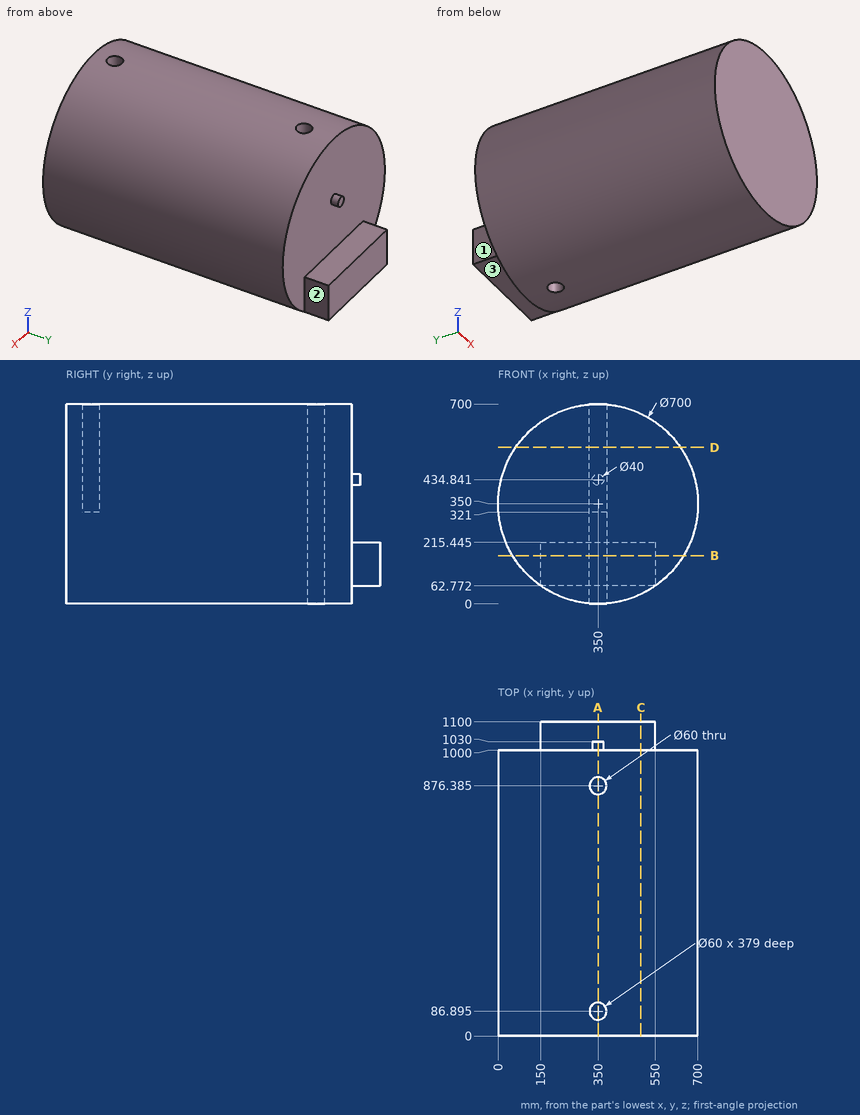
Verification items for this drawing (mm, ordinates from the low corner). A direction names the side the tool comes from. Coordinates: 2 decimals unless noted, no trailing zeros. Write each loop counter-clockwise with the first axis right and the second up, starting at its lowest first coordinate (ties: lowest second). Pieces come first, ordered by that corner, then holes. Notation, with made-up numbers: (-7.75, 54) - (10.25, 54) arc R29 ccw to (10.25, 83) - close; hole circle Ø3 at (-8.5, 31). An arc over 180 degrees is marked (long way). One line per question, with ' | ' between items.
Item 1: Sectioned sample at A-A on x = 350. Record the boundary of the cut face in (y, z) (1 decimal), plus the area to 3 significant figures.
Determined:
outline: (0, 0) - (846.4, 0) - (846.4, 700) - (116.9, 700) - (116.9, 321) - (56.9, 321) - (56.9, 700) - (0, 700) - close; (906.4, 0) - (1000, 0) - (1000, 62.8) - (1100, 62.8) - (1100, 215.4) - (1000, 215.4) - (1000, 414.8) - (1030, 414.8) - (1030, 454.8) - (1000, 454.8) - (1000, 700) - (906.4, 700) - close | area: 652,000 mm2
Item 2: Access from +Z, -Z, +X, -X, +Y, -Y to the whole of each face (thin tool, end or side, straight path). Record for the marked faces 1, 2 and 3.
Determined:
face 1: +Z, -Z, -X, +Y | face 2: +Z, -Z, +X, +Y | face 3: -Z, +X, -X, +Y
Item 3: Sectioned sample at D-D on z = 548. Record the boundary of the cut face in (x, y) (1 decimal), plus the area to 3 significant figures.
Determined:
outline: (61.4, 0) - (638.6, 0) - (638.6, 1000) - (61.4, 1000) - close; hole circle Ø60 at (350, 86.9); hole circle Ø60 at (350, 876.4) | area: 572,000 mm2
Item 4: Sectioned sample at C-C on x = 500. Record the boundary of the cut face in (y, z) (1 decimal).
Determined:
outline: (0, 33.8) - (1000, 33.8) - (1000, 62.8) - (1100, 62.8) - (1100, 215.4) - (1000, 215.4) - (1000, 666.2) - (0, 666.2) - close
Item 5: Sectioned sample at B-B on z = 169. Record the boundary of the cut face in (x, y) (1 decimal).
Determined:
outline: (50.4, 0) - (649.6, 0) - (649.6, 1000) - (550, 1000) - (550, 1100) - (150, 1100) - (150, 1000) - (50.4, 1000) - close; hole circle Ø60 at (350, 876.4)
Item 6: Thickness scan on line 1 (Y direction, x = 350, z = 468) (1 decimal); line 2 (X direction, y = 874, z = 354.5) (1 decimal); line 3 (X direction, y = 892.5, z = 598) (1 decimal). Record the ranges inside material, lowest first. Write a range as [from, to].
Determined:
line 1: y = [0, 56.9], [116.9, 846.4], [906.4, 1000] | line 2: x = [0, 320.1], [379.9, 700] | line 3: x = [103, 324.7], [375.3, 597]
Item 7: Gauge pin test, flat ends, axial feed: P1, Ø6, axis at x = 499, y = 148.5, coming from the +Z side (1 decimal); P2, Ø20, axis at x = 348.5, z = 436, coming from the +Y side; P3, Ø8, axis at x = 157.5, y = 866, coming from the +Z side. Record the tip position at first contact, or that the pin passes through.
Determined:
P1: stops at z = 668.1 | P2: stops at y = 1030 | P3: stops at z = 644.9
